```python
from build123d import *

# Parameters (mm, degrees)
F2_R     = 11.5
F3_DEPTH = 80.518
F5_DEPTH = 40


# Not quite as in the source:
# - ends of sketch curves that miss each other by under 0.0002 mm in the source are joined


with BuildPart() as f1:
    # F0 (on Front) → F1 (revolve)
    with BuildSketch(Plane.XZ):
        Polygon((-30.76, 31.115), (-38.89375, 31.115), (-38.89375, -31.115), (-30.76, -31.115), (30.76, -31.115), (38.89375, -31.115), (38.89375, 31.115), (30.76, 31.115), (25.8486765474, 17.62125), (20.2913232706, 17.62125), (15.379999922, 31.115), (10.4686765734, 17.62125), (4.9113232966, 17.62125), (-5.2e-08, 31.115), (-4.9113234006, 17.62125), (-10.4686766774, 17.62125), (-15.380000026, 31.115), (-20.2913233746, 17.62125), (-25.8486766514, 17.62125), align=None)
    revolve(axis=Axis((0, 0, -31.115), (1, 0, 0)))

    # F2 (on face) → F3 (cut)
    with BuildSketch(Plane.YZ.offset(38.89375)):
        with Locations((0, -31.115)):
            Circle(F2_R)
    extrude(amount=-F3_DEPTH, mode=Mode.SUBTRACT)

    # F4 (on face) → F5 (cut)
    with BuildSketch(Plane.YZ.offset(38.89375)):
        with BuildLine():
            Line((2, -15.615), (0, -15.615))
            Line((0, -15.615), (-2, -15.615))
            Line((-2, -15.615), (-2, -19.7902483471))
            ThreePointArc((-2, -19.7902483471), (0, -19.615), (2, -19.7902483471))
            Line((2, -19.7902483471), (2, -15.615))
        make_face()
    extrude(amount=-F5_DEPTH, mode=Mode.SUBTRACT)


solid = f1.part
```
Could you check a few things on this model? Use its own coordinates, in mm. A direction names the side the tool comes from. Coordinates: 2 decimals unless noted, no trailing zeros. Order: outer loops, then holes, each group sorted by start corner. A loop starts at its lowest first (then second) coordinate and runs counter-clockwise, first axis right, second up. Notation, with made-up numbers: M -17,57.5 L 23,57.5 A16 cw 23,70.5 Z; hole C -30.75,69 d7. An arc over 180 degrees is marked long. Use one line per item in the form item = value. Start each with the question number.
1. Suppose I cut it at A-A on x = 22.5. Write out the boundary of the cut face in (y, z) (1 decimal).
2. We'd pull the mould along X, two halves only. Please class faces 4 (the flat face through (19, 2, -18)), 5 (the flat face through (-1.106, 0, -18)), 6 (the cylindrical face through (-23.109, 29.655, -69.79)): +X half, -X half, draft (parallel to the pull), parting line (faces both ways), or undercut.
3. For pin 1 (8 mm diameter, centred on x = -19, y = -39.5, fed in from +Z); pin 2 (18.5 mm diameter, centred on y = 0, z = -31.115, fed in from +X); pin 3 (3 mm diameter, centred on x = -22.5, z = 1, fed in from -Y); pin 4 (1.5 mm diameter, centred on x = 24, y = 37.5, fed in from +Z), each with a flat end and sliding along its axis, tell me the tip position at first contact or that it passes through.
4. On a 3-axis mill with a long thin cutter (end or side, diameter ignored), from which of +Z, -Z, +X, -X, +Y, -Y can I reach the whole of each face in a straight line? I mean faces 1 (the conical face through (19.984, 48.401, -41.863)), 2 (the flat face through (38.894, -1, -44)), 3 (the flat face through (19, 0, -15.615)). Say none if no direction works.
5. Please list where these lines run through material, in increasing order: line 1 (X direction, y = 43.5, z = -7.5); line 2 (X direction, y = -52, z = 0.5); line 3 (Z direction, x = -8, y = 0) (3 decimals).
6. Suppose I cut it at B-B on z = 23. Count the separate pieces of the cut face and the enclosed holes in it, then the cut area to 3 significant figures.
7. Suppose I cut it at C-C on x = -18.5. Write out the boundary of the cut face in (y, z) (3 decimals), then the cut area to 3 significant figures.
Geometry says:
q1.outline = C 0,-31.1 d97.5; hole M -2,-19.8 A11.5 ccw long 2,-19.8 L 2,-15.6 L -2,-15.6 Z
q2.face_4 = draft
q2.face_5 = +X half
q2.face_6 = undercut
q3.pin_1 = 18.32
q3.pin_2 = through
q3.pin_3 = -37.92
q3.pin_4 = 0.9
q4.face_1 = none
q4.face_2 = +Z, -Z, +X, +Y, -Y
q4.face_3 = +X
q5.line_1 = -38.89 to -26.13, -20.01 to -10.75, -4.63 to 4.63, 10.75 to 20.01, 26.13 to 38.89
q5.line_2 = -38.89 to -30.26, -15.88 to -14.88, -0.5 to 0.5, 14.88 to 15.88, 30.26 to 38.89
q5.line_3 = -79.851 to -42.615, -19.615 to 17.621
q6.separate_pieces = 5
q6.enclosed_holes = 0
q6.area = 1,950 mm^2
q7.outline = C 0,-31.115 d107.316; hole C 0,-31.115 d23
q7.area = 8,630 mm^2
